The figure shows three views and two pictorial views of one solid part (mm, origin at its lowest corner). Answer the questions. Give positions to 0.01 mm unless a question says otherwise; leave off trailing zeros. Loops run counter-clockwise (first coordinate to the right, second up) from the corner with the lowest first, then second, coordinate; pieces in that order, holes last. Notation, with made-up numbers: (46, -31.75) -> (94, -31.75) arc R14 cw to (94, -5.75) -> close; hole circle Ø4 at (49.5, 66). An arc over 180 degrees is marked (long way). One line per item, written item: value. Start each with the question number.
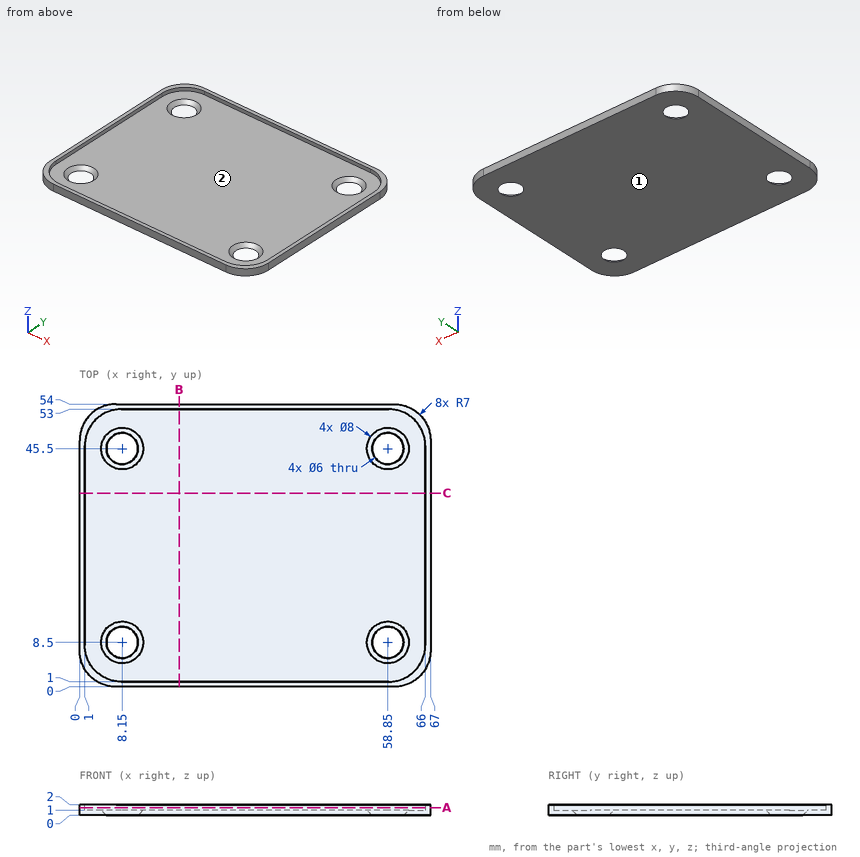
Item 1: Consider L1, parallel to X at y = 40, z = 1.6; L2, parallel to X at y = 8.5, z = 0.05; L3, parallel to Y at x = 45, z = 1.85. Determine where each line is inside the solid, lowest interval first. Write a range as [from, to].
Item 2: Section B-B, the plane x = 19 is taken. Determine the outline of the cut face in (y, z), plus the area to 3 significant figures.
Item 3: Section C-C, the plane y = 37 is taken. Determine the outline of the cut face in (x, z).
Item 4: Section A-A, the plane z = 1.5 is taken. Determine the outline of the cut face in (x, y).
Item 5: Flat-ended cylindrical pins translate along their axes: pin 1 (1 mm diameter, centred on y = 27.5, z = 0.5, fed in from -X); pin 2 (8 mm diameter, centred on x = 58.5, y = 28.5, fed in from +Z); pin 3 (5 mm diameter, centred on x = 8.15, y = 8.5, fed in from -Z); pin 4 (7 mm diameter, centred on x = 58.85, y = 8.5, fed in from +Z). Find the tip coordinate at first contact, or state that the pin passes through.
Item 6: Determine the mould class of the marked faces 1 and 2 for opening direction X: pulls with the +X half, pulls with the -X half, needs draft (parallel to the pull), parting line crosses it, or undercut.
Computed values:
1. L1: [0, 1], [66, 67]
1. L2: [0, 5.1], [11.2, 55.8], [61.9, 67]
1. L3: [0, 1], [53, 54]
2. outline: (0, 0) -> (54, 0) -> (54, 2) -> (53, 2) -> (53, 1) -> (1, 1) -> (1, 2) -> (0, 2) -> close
2. area: 56.0 mm²
3. outline: (0, 0) -> (67, 0) -> (67, 2) -> (66, 2) -> (66, 1) -> (1, 1) -> (1, 2) -> (0, 2) -> close
4. outline: (0, 7) arc R7 ccw to (7, 0) -> (60, 0) arc R7 ccw to (67, 7) -> (67, 47) arc R7 ccw to (60, 54) -> (7, 54) arc R7 ccw to (0, 47) -> close; hole (1, 8) arc R7 ccw to (8, 1) -> (59, 1) arc R7 ccw to (66, 8) -> (66, 46) arc R7 ccw to (59, 53) -> (8, 53) arc R7 ccw to (1, 46) -> close
5. pin 1: x = 0
5. pin 2: z = 1
5. pin 3: through
5. pin 4: z = 0.5
6. face 1: needs draft
6. face 2: undercut
